from build123d import *

# Parameters (mm, degrees)
F1_DEPTH = 30
F2_DEPTH = 20
F4_DEPTH = 10
F5_SIZE  = 5
F6_W     = 31.7785144259
F6_H     = 10.2327512205
F6_H_2   = 5
F7_DEPTH = 8
F8_SIZE  = 5


with BuildPart() as f1:
    # F0 (on Top) → F1 (new body)
    with BuildSketch(Plane.XY):
        with BuildLine():
            ThreePointArc((15.9804643873, 2.9474154722), (16.182475804, 1.4798570381), (16.25, 0))
            ThreePointArc((16.25, 0), (2.1533060737, -16.1066996294), (-15.6793259019, -4.2686343556))
            Line((-15.6793259019, -4.2686343556), (-17.3869081956, -4.6578346252))
            ThreePointArc((-17.3869081956, -4.6578346252), (2.3490053723, -17.8460688601), (18, 0))
            ThreePointArc((18, 0), (17.9218419848, 1.6755834418), (17.6880466811, 3.3366157419))
            Line((17.6880466811, 3.3366157419), (15.9804643873, 2.9474154722))
        make_face()
    extrude(amount=F1_DEPTH)

    # F0 (on Top) → F2 (join)
    with BuildSketch(Plane.XY):
        with BuildLine():
            ThreePointArc((15.9804643873, 2.9474154722), (16.182475804, 1.4798570381), (16.25, 0))
            ThreePointArc((16.25, 0), (2.1533060737, -16.1066996294), (-15.6793259019, -4.2686343556))
            Line((-15.6793259019, -4.2686343556), (-17.3869081956, -4.6578346252))
            ThreePointArc((-17.3869081956, -4.6578346252), (2.3490053723, -17.8460688601), (18, 0))
            ThreePointArc((18, 0), (17.9218419848, 1.6755834418), (17.6880466811, 3.3366157419))
            Line((17.6880466811, 3.3366157419), (15.9804643873, 2.9474154722))
        make_face()
        with BuildLine():
            ThreePointArc((-15.6793259019, -4.2686343556), (-3.6111653073, 15.8436733469), (15.9804643873, 2.9474154722))
            Line((15.9804643873, 2.9474154722), (17.6880466811, 3.3366157419))
            ThreePointArc((17.6880466811, 3.3366157419), (-4.0000600327, 17.549915092), (-17.3869081956, -4.6578346252))
            Line((-17.3869081956, -4.6578346252), (-15.6793259019, -4.2686343556))
        make_face()
    extrude(amount=F2_DEPTH)

    # F3 (on face) → F4 (join)
    with BuildSketch(Plane.XY.offset(30)):
        with BuildLine():
            ThreePointArc((15.9804643873, 2.9474154722), (3.6111653073, -15.8436733469), (-15.6793259019, -4.2686343556))
            Line((-15.6793259019, -4.2686343556), (-17.3869081956, -4.6578346252))
            ThreePointArc((-17.3869081956, -4.6578346252), (4.0000600327, -17.549915092), (17.6880466811, 3.3366157419))
            Line((17.6880466811, 3.3366157419), (15.9804643873, 2.9474154722))
        make_face()
        with BuildLine():
            Line((-17.3869081956, -4.6578346252), (-15.6793259019, -4.2686343556))
            ThreePointArc((-15.6793259019, -4.2686343556), (3.6111653073, -15.8436733469), (15.9804643873, 2.9474154722))
            Line((15.9804643873, 2.9474154722), (17.6880466811, 3.3366157419))
            ThreePointArc((17.6880466811, 3.3366157419), (16.2041492949, 7.8374450957), (13.5969934668, 11.7949891337))
            Line((13.5969934668, 11.7949891337), (-17.3652541608, 4.7379265435))
            ThreePointArc((-17.3652541608, 4.7379265435), (-17.3761273243, 4.6978930607), (-17.3869081956, 4.6578346252))
            ThreePointArc((-17.3869081956, 4.6578346252), (-17.9872433705, 0.6775514234), (-17.6880466811, -3.3366157419))
            Line((-17.6880466811, -3.3366157419), (-17.3869081956, -4.6578346252))
        make_face()
        with BuildLine():
            Line((-17.3869081956, 4.732991053), (-17.3869081956, 4.6578346252))
            ThreePointArc((-17.3869081956, 4.6578346252), (-17.3761273243, 4.6978930607), (-17.3652541608, 4.7379265435))
            Line((-17.3652541608, 4.7379265435), (-17.3869081956, 4.732991053))
        make_face()
    extrude(amount=F4_DEPTH)

    # F5
    f5_edges = [f1.edges().sort_by_distance(p)[0] for p in [
        (-1.894957, 8.26399, 30),
    ]]
    chamfer(f5_edges, length=F5_SIZE)

    # F6 (on face) → F7 (join)
    with BuildSketch(Plane(origin=(-1.884130347, 8.2664578386, 0), x_dir=(-0.9749952829, -0.2222255574, 0), z_dir=(-0.2222255574, 0.9749952829, 0))):
        with Locations((0.011104687, 34.8836243898)):
            Rectangle(F6_W, F6_H)
        with Locations((0.011104687, 37.5)):
            Rectangle(F6_W, F6_H_2)
    extrude(amount=F7_DEPTH)

    # F8
    f8_edges = [f1.edges().sort_by_distance(p)[0] for p in [
        (-1.894957, 8.26399, 29.767249),
    ]]
    chamfer(f8_edges, length=F8_SIZE)


solid = f1.part
Could you check a few things on this model? Use its own coordinates, in mm. A direction names the side the tool comes from. Coordinates: 2 decimals unless noted, no trailing zeros. Write each loop counter-clockwise with the first axis right and the second up, starting at its lowest first coordinate (ties: lowest second). Pieces come first, ordered by that corner, then holes. Notation, with made-up numbers: (82.5, 28) - (107.5, 28) arc R24 cw to (107.5, 62) - close; hole circle Ø9 at (42, -6). An arc over 180 degrees is marked (long way). Write item = value, one per line.
1) Suppose I cut it at C-C on y = 6. Please give me the cut outline in (x, z), plus the area to 3 significant figures.
Result set:
outline = (-17.68, 33.47) - (-11.83, 34.77) - (-11.83, 35) - (10.67, 30) - (16.97, 30) - (16.97, 40) - (-17.68, 40) - close; (-16.97, 0) - (-15.1, 0) - (-15.1, 20) - (-16.97, 20) - close; (15.1, 0) - (16.97, 0) - (16.97, 20) - (15.1, 20) - close
area = 341 mm2
2) Suppose I cut it at D-D on z = 37.5. Please give me the cut outline in (x, y).
Result set:
outline = (-19.16, 12.53) - (-17.39, 4.73) - (-17.39, 4.66) arc R18 ccw to (-17.69, -3.34) - (-17.39, -4.66) arc R18 ccw (long way) to (13.6, 11.79) - (11.82, 19.59) - close
3) Will these pins go through, and if not, where does the flat tip stop? pin 1 Ø3 at (y, z) = (-4, 30) entering from +X; pin 2 Ø1.5 at (y, z) = (-9, 24) entering from -X; pin 3 Ø8 at (x, y) = (-14.5, -0.5) entering from -Z; pin 4 Ø8 at (y, z) = (-14, 12) entering from +X.
Result set:
pin_1 = 17.83
pin_2 = -16
pin_3 = 0
pin_4 = 14.97
4) Suppose I cut it at A-A on z = 17.5. Please give me the cut outline in (x, y).
Result set:
outline = circle Ø36 at (0, 0); hole circle Ø32.5 at (0, 0)
5) Please list where these lines run through material, in increasing order: line 1 (Z direction, x = 5, y = 17); line 2 (Z direction, x = 7, y = -8.5); line 3 (Z direction, x = 6, y = 17.5). Write a range as [from, to].
Result set:
line_1 = [0, 20], [29.77, 40]
line_2 = [30, 40]
line_3 = [29.77, 40]
6) We'd pull the mould along Y, two halves only. Please class faces 1 (the flat face through (-18.263, 8.578, 35.949)), 2 (the flat face through (-3.456, 16.113, 34.955)), 3 (the flat face through (-4, 16, 0)): +Y half, -Y half, draft (parallel to the pull), parting line (faces both ways), or undercut.
Result set:
face_1 = undercut
face_2 = +Y half
face_3 = draft
7) For faces 4 (the flat face through (-2.23, 10.72, 32.3)), 5 (the cylindrical face through (-17.985, 0.734, 36.041)), 6 (the flat face through (-3, 15, 29.767)), 7 (the flat face through (-4, 16, 20)), which set-ups out of +Z, -Z, +X, -X, +Y, -Y let a thin tool reach every point of the face, with its end or its side?
Result set:
face_4 = none
face_5 = +Z, -Z, -X
face_6 = +X, -X, +Y
face_7 = -X, +Y
8) Suppose I cut it at B-B on x = -9.5. Please give me the cut outline in (y, z), plus the area to 3 significant figures.
Result set:
outline = (-15.29, 0) - (-13.18, 0) - (-13.18, 30) - (1.4, 30) - (6.53, 35) - (6.53, 34.77) - (11.66, 29.77) - (14.74, 29.77) - (14.74, 40) - (-15.29, 40) - close; (13.18, 0) - (15.29, 0) - (15.29, 20) - (13.18, 20) - close
area = 382 mm2
